Print and shaded views of the part. All mm, measured from the part's lowest x, y and z. A direction names the side the tool comes from. Round coordinates to 2 decimals unless told otherwise and drop trailing zeros. Order: outer loops, then holes, each group sorted by start corner. A loop starts at its lowest first (then second) coordinate and runs counter-clockwise, first axis right, second up. Notation, with made-up numbers: (23.25, 42.5) -> (32.25, 42.5) arc R22 cw to (32.25, 76.5) -> close; hole circle Ø8 at (-15, 84). An arc over 180 degrees is marked (long way). Answer as CSV lines item,"result".
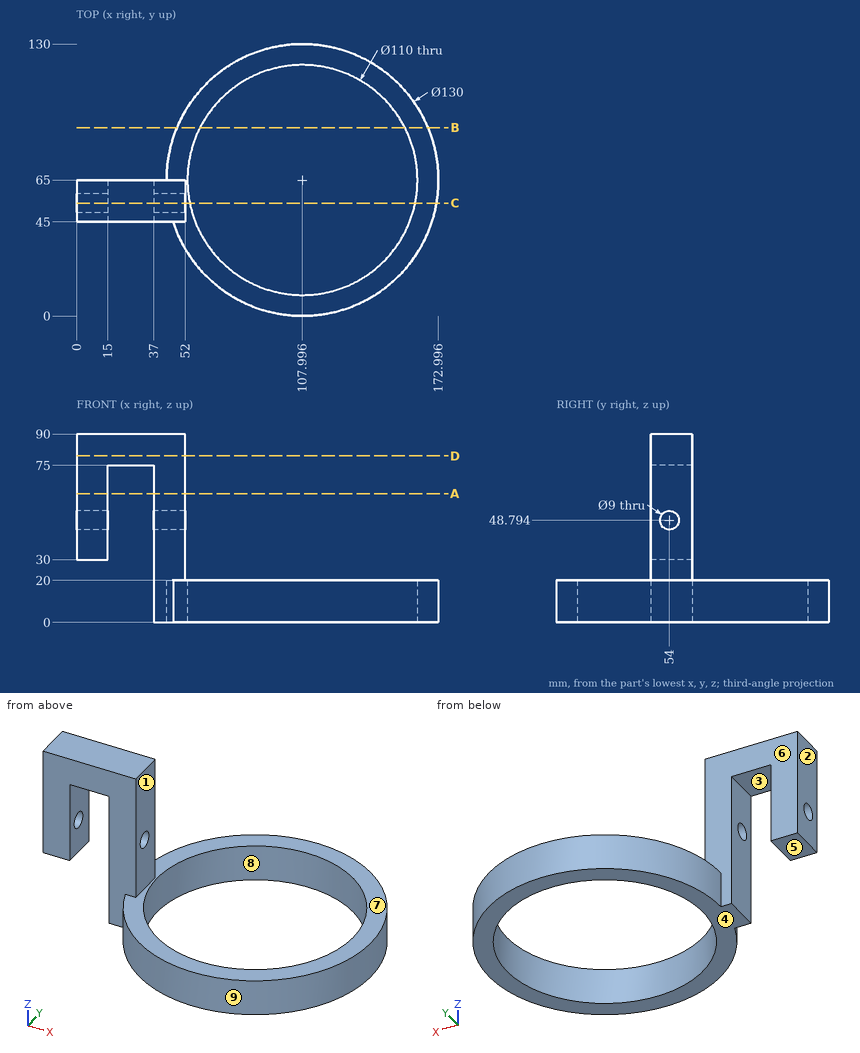
Q1. Saw through at A-A (z = 61.5). Write the cut outline in (x, y), plus the area to 3 significant figures.
Checks:
outline,"(0, 45) -> (15, 45) -> (15, 65) -> (0, 65) -> close; (37, 45) -> (52, 45) -> (52, 65) -> (37, 65) -> close"
area,"600 mm²"
Q2. Saw through at D-D (z = 79.5). Write the cut outline in (x, y).
Checks:
outline,"(0, 45) -> (52, 45) -> (52, 65) -> (0, 65) -> close"
Q3. Mould opens along Y. For the marked faces 6, 7, 8 and 9 say: +Y half, -Y half, draft (parallel to the pull), parting line (faces both ways), or undercut.
Checks:
face 6,"+Y half"
face 7,"draft"
face 8,"undercut"
face 9,"parting line"
Q4. Tool access for the marked faces 1, 2, 3, 4 and 5: list every direction of +Z, -Z, +X, -X, +Y, -Y with a clear straight run to the whole face (end or side of a thin tool).
Checks:
face 1,"+Z, +X, +Y, -Y"
face 2,"+Z, -Z, -X, +Y, -Y"
face 3,"-Z, +Y, -Y"
face 4,"-Z, +X, -X, +Y, -Y"
face 5,"-Z, -X, +Y, -Y"
Q5. Saw through at C-C (y = 54). Write the cut outline in (x, z) (1 decimal).
Checks:
outline,"(0, 30) -> (15, 30) -> (15, 44.3) -> (0, 44.3) -> close; (0, 53.3) -> (15, 53.3) -> (15, 75) -> (37, 75) -> (37, 53.3) -> (52, 53.3) -> (52, 90) -> (0, 90) -> close; (37, 0) -> (54.1, 0) -> (54.1, 20) -> (52, 20) -> (52, 44.3) -> (37, 44.3) -> close; (161.9, 0) -> (172.1, 0) -> (172.1, 20) -> (161.9, 20) -> close"
Q6. Saw through at B-B (y = 90). Write the cut outline in (x, z) (1 decimal).
Checks:
outline,"(48, 0) -> (59, 0) -> (59, 20) -> (48, 20) -> close; (157, 0) -> (168, 0) -> (168, 20) -> (157, 20) -> close"
Q7. Flat gauge pins, fed straight in: pin 1 (16 mm diameter, centred on y = 53.5, z = 50, fed in from +X); pin 2 (16 mm diameter, centred on x = 26, y = 52, fed in from -Z); pin 3 (4.5 mm diameter, centred on x = 6.5, y = 50.5, fed in from -Z). Where does each tip first touch, or does it go through?
Checks:
pin 1,"x = 52"
pin 2,"z = 75"
pin 3,"z = 30"
Q8. Wall check: L1, parallel to X at y = 47, z = 35.5; L2, parallel to Z at x = 8, y = 54; L3, parallel to X at y = 100, z = 11 (1 decimal). Give the ranges that are in metal, low to high. Write a range as [from, to].
Checks:
L1,"[0, 15], [37, 52]"
L2,"[30, 44.29], [53.29, 90]"
L3,"[53.2, 65.6], [150.4, 162.8]"
